Check sheet for the modelled part. Datum: model origin and axes. Units: mm. A direction names the side the tool comes from. Round coordinates to 2 decimals unless told otherwise and drop trailing zeros. Order: outer loops, then holes, each group sorted by start corner. A loop starts at its lowest first (then second) coordinate and runs counter-clockwise, first axis right, second up. Notation, with made-up numbers: (45.25, 79) -> (81.25, 79) arc R14 cw to (81.25, 85) -> close; hole circle Ø5 at (49, 52.25). An arc over 180 degrees is marked (long way). Answer in a Markdown table with one row per item.
Autodesk Inventor part; units mm, degrees
ref_plane "YZ Plane" through (0, 0, 0) normal (1, 0, 0) x (0, 1, 0)
ref_plane "XZ Plane" through (0, 0, 0) normal (0, 1, 0) x (-1, 0, 0)
ref_plane "XY Plane" through (0, 0, 0) normal (0, 0, 1) x (1, 0, 0)
sketch "Skizze1" plane through (0, 0, 0) normal (0, 0, 1) x (1, 0, 0)
  line L0 (-160.1182, 0) -> (119.8818, 0)
  line L1 (0, -160.7697) -> (0, 119.2303)
  line L2 (-120.1182, 79.2303) -> (79.8818, 79.2303)
  line L3 (79.8818, 79.2303) -> (79.8818, -120.7697)
  line L4 (79.8818, -120.7697) -> (-120.1182, -120.7697)
  line L5 (-120.1182, -120.7697) -> (-120.1182, 79.2303)
  line L6 (-110.1182, 69.2303) -> (69.8818, 69.2303)
  line L7 (69.8818, 69.2303) -> (69.8818, -110.7697)
  line L8 (69.8818, -110.7697) -> (-110.1182, -110.7697)
  line L9 (-110.1182, -110.7697) -> (-110.1182, 69.2303)
  point P0 (0, 0)
  dimension "d0" = 200
  dimension "d1" = 200
  dimension "d2" = 10
  dimension "d3" = 10
  dimension "d4" = 10
  dimension "d5" = 10
extrude "Extrusion1" add sketch "Skizze1" along normal blind 150 contours L5 L2 L1 L6 L9 L0 | L0 L9 L8 L1 L4 L5 | L1 L8 L7 L0 L3 L4 | L2 L3 L0 L7 L6 L1
sketch "Skizze2" plane through (-120.1182, -120.7697, 0) normal (-1, 0, 0) x (0, 0, 1)
  point P0 (0, 120.7697)
sketch "Skizze3" plane through (-120.1182, -120.7697, 0) normal (-1, 0, 0) x (0, 0, 1)
  point P0 (0, 120.7697)
sketch "Skizze4" plane through (-120.1182, -120.7697, 0) normal (-1, 0, 0) x (0, 0, 1)
  point P0 (0, 120.7697)
sketch "Skizze5" plane through (-120.1182, -120.7697, 0) normal (-1, 0, 0) x (0, 0, 1)
  point P0 (0, 120.7697)
sketch "Skizze6" plane through (-120.1182, -120.7697, 0) normal (-1, 0, 0) x (0, 0, 1)
  point P0 (0, 120.7697)
sketch "Skizze7" plane through (0, 0, 0) normal (0, 0, -1) x (-1, 0, 0)
  line L0 (120.1182, 79.2303) -> (120.1182, -120.7697)
  line L1 (120.1182, 79.2303) -> (170.1182, 79.2303)
  line L2 (170.1182, -120.7697) -> (120.1182, -120.7697)
  line L3 (120.1182, -120.7697) -> (120.1182, 79.2303)
  arc A0 (170.1182, -120.7697) -> (170.1182, 79.2303) centre (170.1182, -20.7697) ccw
  line L4 (120.1182, 69.2303) -> (162.1378, 69.2303)
  line L5 (162.1378, -110.7697) -> (120.1182, -110.7697)
  line L6 (120.1182, -110.7697) -> (120.1182, 69.2303)
  arc A1 (162.1378, -110.7697) -> (162.1378, 69.2303) centre (162.1378, -20.7697) ccw
  point P0 (0, 0)
  dimension "d9" = 10
  dimension "d10" = 10
extrude "Extrusion2" add sketch "Skizze7" against normal blind 150 contours L1 A0 L2 L0 L5 A1 L4
sketch "Skizze8" plane through (-110.1182, -110.7697, 0) normal (1, 0, 0) x (0, 0, -1)
  line L0 (-150, 0) -> (-150, 180)
  line L1 (0, 0) -> (0, 180)
  line L2 (-150, 0) -> (0, 0)
  line L3 (0, 0) -> (0, 180)
  line L4 (0, 180) -> (-150, 180)
  line L5 (-150, 180) -> (-150, 0)
  point P0 (0, 110.7697)
extrude "Extrusion3" add sketch "Skizze8" along normal blind 10
sketch "Skizze9" plane through (0, 0, 0) normal (0, 0, -1) x (-1, 0, 0)
  line L0 (-79.8818, 79.2303) -> (170.1182, 79.2303)
  line L1 (-79.8818, 79.2303) -> (120.1182, 79.2303)
  line L2 (120.1182, 79.2303) -> (120.1182, -110.7697)
  line L3 (120.1182, -110.7697) -> (-79.8818, -110.7697)
  line L4 (-79.8818, -110.7697) -> (-79.8818, 79.2303)
  arc A0 (170.1182, -120.7697) -> (170.1182, 79.2303) centre (170.1182, -20.7697) ccw
  arc A1 (170.1182, -120.7697) -> (170.1182, 79.2303) centre (170.1182, -20.7697) ccw
  line L5 (120.1182, 79.2303) -> (170.1182, 79.2303)
  line L6 (-79.8818, -120.7697) -> (170.1182, -120.7697)
  line L7 (120.1182, -120.7697) -> (170.1182, -120.7697)
  line L8 (120.1182, -110.7697) -> (-79.8818, -110.7697)
  line L9 (-79.8818, -110.7697) -> (-79.8818, -120.7697)
  line L10 (-79.8818, -120.7697) -> (120.1182, -120.7697)
  line L11 (120.1182, -120.7697) -> (120.1182, -110.7697)
  point P0 (0, 0)
  point P1 (-79.8818, -110.7697)
extrude "Extrusion4" add sketch "Skizze9" along normal blind 10
sketch "Skizze10" plane through (0, 0, 150) normal (0, 0, 1) x (1, 0, 0)
  point P0 (0, 0)
sketch "Skizze11" plane through (0, 0, 150) normal (0, 0, 1) x (1, 0, 0)
  line L0 (-107.6182, 76.7303) -> (77.3818, 76.7303)
  line L1 (77.3818, 76.7303) -> (77.3818, 71.09)
  line L2 (72.3818, 71.7303) -> (-102.6182, 71.7303)
  line L3 (-107.6182, 71.09) -> (-107.6182, 76.7303)
  line L4 (77.3818, -113.2626) -> (77.3818, -118.2697)
  line L5 (77.3818, -118.2697) -> (-107.6182, -118.2697)
  line L6 (-107.6182, -118.2697) -> (-107.6182, -113.2626)
  line L7 (77.3818, -113.2626) -> (77.3818, 71.09)
  line L8 (72.3818, 71.7303) -> (72.3818, -113.2697)
  line L9 (-102.6182, 71.7303) -> (-102.6182, -113.2697)
  line L10 (-107.6182, -113.2626) -> (-107.6182, 71.09)
  line L11 (-107.6182, -113.2626) -> (-107.6182, -113.2626)
  line L12 (-102.6182, -113.2697) -> (72.3818, -113.2697)
  line L13 (77.3818, -113.2626) -> (77.3818, -113.2626)
  line L14 (79.8818, 79.2303) -> (-170.1182, 79.2303)
  line L15 (79.8818, -120.7697) -> (79.8818, 79.2303)
  line L16 (-100.1182, 69.2303) -> (69.8818, 69.2303)
  line L17 (69.8818, 69.2303) -> (69.8818, -110.7697)
  line L18 (69.8818, -110.7697) -> (-100.1182, -110.7697)
  line L19 (-170.1182, -120.7697) -> (79.8818, -120.7697)
  line L20 (-100.1182, 69.2303) -> (-100.1182, -110.7697)
  point P0 (0, 0)
  dimension "d17" = 2.5
  dimension "d18" = 2.5
  dimension "d19" = 2.5
  dimension "d20" = 2.5
  dimension "d21" = 2.5
  dimension "d22" = 2.5
  dimension "d23" = 2.5
  dimension "d24" = 2.5
  dimension "d25" = 5
  dimension "d26" = 5
extrude "Extrusion5" cut sketch "Skizze11" against normal blind 5 contours L0 L1 L7 L4 L5 L6 L10 L3
sketch "Skizze12" plane through (0, 0, 0) normal (0, 0, 1) x (1, 0, 0)
  line L0 (-100.1182, 69.2303) -> (69.8818, 69.2303)
  line L1 (69.8818, 69.2303) -> (69.8818, -110.7697)
  line L2 (-20.1182, -15.7697) -> (-10.1182, -15.7697)
  line L3 (-10.1182, -15.7697) -> (-10.1182, -25.7697)
  line L4 (-10.1182, -25.7697) -> (-20.1182, -25.7697)
  line L5 (-20.1182, -25.7697) -> (-20.1182, -15.7697)
  point P0 (0, 0)
  point P1 (-15.1182, -20.7697)
  dimension "d29" = 90
  dimension "d30" = 85
  dimension "d31" = 5
  dimension "d32" = 5
  dimension "d33" = 5
  dimension "d34" = 5
extrude "Extrusion6" cut sketch "Skizze12" against normal blind 5
properties part number "BetterPrototyp"
(1) Depth check by flat-ended pin: pin 1 Ø3 at (y, z) = (-62.5, 81.5) entering from -X; pin 2 Ø2 at (y, z) = (-33, 131.5) entering from -X. Enter the tip coordinate at first touch or a pass-through.
Solutions:
| item | result |
|---|---|
| pin 1 | x = -261.67 |
| pin 2 | x = -269.49 |
(2) Section check A-A on z = 37. Record the boundary of the cut face in (x, y), plus the area to 3 significant figures.
Solutions:
| item | result |
|---|---|
| outline | (-170.12, -120.77) -> (79.88, -120.77) -> (79.88, 79.23) -> (-170.12, 79.23) arc R100 ccw to start; hole (-162.14, -110.77) -> (-120.12, -110.77) -> (-120.12, 69.23) -> (-162.14, 69.23) arc R90 ccw to start; hole (-100.12, -110.77) -> (69.88, -110.77) -> (69.88, 69.23) -> (-100.12, 69.23) -> close |
| area | 14,800 mm^2 |
(3) Section check B-B on x = -34. Record the boundary of the cut face in (y, z).
Solutions:
| item | result |
|---|---|
| outline | (-120.77, -10) -> (79.23, -10) -> (79.23, 150) -> (76.73, 150) -> (76.73, 145) -> (71.73, 145) -> (71.73, 150) -> (69.23, 150) -> (69.23, 0) -> (-110.77, 0) -> (-110.77, 150) -> (-113.27, 150) -> (-113.27, 145) -> (-118.27, 145) -> (-118.27, 150) -> (-120.77, 150) -> close |
(4) Draft check along Y on faces 1 (the flat face through (-43, 79.23, 69)), 2 (the flat face through (-141, -110.77, 74)), 3 (the flat face through (-47, -120.77, 69)). Enter one of: pulls with the +Y half, pulls with the -Y half, needs draft (parallel to the pull), parting line crosses it, or undercut.
Solutions:
| item | result |
|---|---|
| face 1 | pulls with the +Y half |
| face 2 | undercut |
| face 3 | pulls with the -Y half |
(5) Tool access check on faces 4 (the cylindrical face through (-270.094, -22.969, 68.88)), 5 (the flat face through (-171, -20, 0)). Record the directions out of +Z, -Z, +X, -X, +Y, -Y that give a thin tool (end or side, any length) a straight path to the whole face; none if there is none.
Solutions:
| item | result |
|---|---|
| face 4 | +Z, -Z, -X |
| face 5 | +Z |
(6) Section check C-C on y = -42.5. Record the boundary of the cut face in (x, z).
Solutions:
| item | result |
|---|---|
| outline | (-267.73, -10) -> (79.88, -10) -> (79.88, 150) -> (77.38, 150) -> (77.38, 145) -> (72.38, 145) -> (72.38, 150) -> (69.88, 150) -> (69.88, 0) -> (-100.12, 0) -> (-100.12, 150) -> (-102.62, 150) -> (-102.62, 145) -> (-107.62, 145) -> (-107.62, 150) -> (-120.12, 150) -> (-120.12, 0) -> (-249.48, 0) -> (-249.48, 150) -> (-267.73, 150) -> close |
(7) Section check D-D on x = -186.5. Record the boundary of the cut face in (y, z), plus the area to 3 significant figures.
Solutions:
| item | result |
|---|---|
| outline | (-119.42, -10) -> (77.88, -10) -> (77.88, 150) -> (65.87, 150) -> (65.87, 0) -> (-107.41, 0) -> (-107.41, 150) -> (-119.42, 150) -> close |
| area | 5,580 mm^2 |
(8) Scan lines: probe 1 along X at (y, z) = (-24, 47); probe 2 along Y at (x, z) = (-49, 34); probe 3 along X at (y, z) = (-100.5, 55). Record each from-to range of solid material in increasing order. Write a range as from..to.
Solutions:
| item | result |
|---|---|
| probe 1 | -270.07..-252.08, -120.12..-100.12, 69.88..79.88 |
| probe 2 | -120.77..-110.77, 69.23..79.23 |
| probe 3 | -230.48..-203.89, -120.12..-100.12, 69.88..79.88 |
